```python
from build123d import *

# Parameters (mm, degrees)
F0_R     = 12.7
F0_R_2   = 10.16
F1_DEPTH = 20.32
F2_DEPTH = 20.32
F3_R     = 9.652
F4_DEPTH = 12.7


with BuildPart() as f1:
    # F0 (on Top) → F1 (new body)
    with BuildSketch(Plane.XY):
        with Locations((-39.235822, 31.019291)):
            Circle(F0_R)
        with Locations((-39.235822, 31.019291)):
            Circle(F0_R_2, mode=Mode.SUBTRACT)
    extrude(amount=F1_DEPTH)

    # F0 (on Top) → F2 (join)
    with BuildSketch(Plane.XY):
        with Locations((-39.235822, 31.019291)):
            Circle(F0_R_2)
        Polygon((-40.496945, 38.614266), (-33.288942, 35.908943), (-32.027819, 28.313968), (-37.974699, 23.424316), (-45.182701, 26.129639), (-46.443824, 33.724614), align=None, mode=Mode.SUBTRACT)
    extrude(amount=F2_DEPTH)

    # F3 (on face) → F4 (cut)
    with BuildSketch(Plane(origin=(0, 0, 0), x_dir=(1, 0, 0), z_dir=(0, 0, -1))):
        with Locations((-39.235822, -31.019291)):
            Circle(F3_R)
    extrude(amount=-F4_DEPTH, mode=Mode.SUBTRACT)


solid = f1.part
```
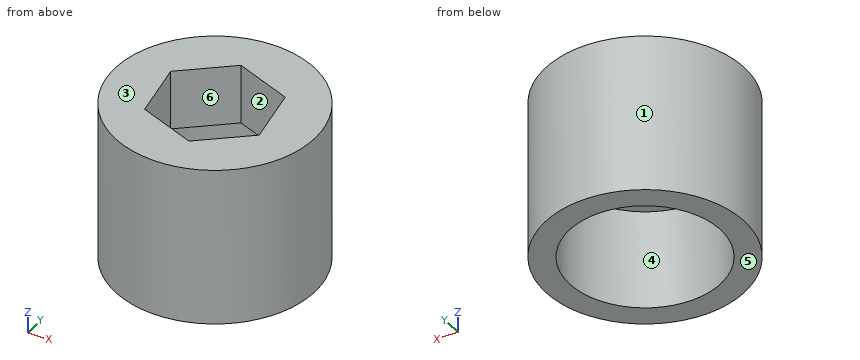
Input: part model. Units: mm. Frame: model coordinates. Face numbers are marked on the shaded views. A direction names the side the tool comes from. Coordinates: 2 decimals unless noted, no trailing zeros. Write each loop counter-clockwise with the first axis right and the second up, starting at its lowest first coordinate (ties: lowest second). Pieces come first, ordered by that corner, then holes. Notation, with made-up numbers: (0, -12) - (14, -12) arc R27 ccw to (14, 8) - close; hole circle Ø10 at (20.25, -39.75). An arc over 180 degrees is marked (long way). Put each result on its own line as item: value. Start each with the question number.
1) Cut plane B-B (x = -37). Return the cut outline in (y, z), plus the area to 3 significant figures.
2) Ray query, L1, parallel to X at y = 25.5, z = 7.25; L2, parallel to Y at x = -39, z = 12.75; L3, parallel to X at y = 33.25, z = 1. Return the intervals inside material, ascending.
3) Cut plane A-A (y = 30.5). Return the cut outline in (x, z), plus the area to 3 significant figures.
4) Cut plane D-D (y = 22.75). Return the cut outline in (x, z).
5) Mould query, pull axis Y, two halves, no side actions, for the marked faces 1, 2 and 3. Classes: pulls with the +Y half, pulls with the -Y half, needs draft (parallel to the pull), parting line crosses it, or undercut.
6) Cut plane C-C (z = 1.75). Return the cut outline in (x, y).
7) Contact query for flat-ended pins moving along their axis: pin 1 (1.5 mm diameter, centred on x = -32, z = 17.5, fed in from -Y); pin 2 (2 mm diameter, centred on y = 22, z = 5.5, fed in from +X); pin 3 (2 mm diameter, centred on x = -41.5, z = 14, fed in from +Y). Output: stop coordinate, or through.
8) Reachability of the marked faces 4, 5 and 6 from +Z, -Z, +X, -X, +Y, -Y: full face, straight path, thin tool, end or side. Return the list, or none.
Resolved:
1. outline: (18.52, 0) - (21.63, 0) - (21.63, 12.7) - (24.23, 12.7) - (24.23, 20.32) - (18.52, 20.32) - close; (37.3, 12.7) - (40.41, 12.7) - (40.41, 0) - (43.52, 0) - (43.52, 20.32) - (37.3, 20.32) - close
1. area: 170 mm2
2. L1: x = -50.67 to -47.15, -31.32 to -27.8
2. L2: y = 18.32 to 23.81, 38.05 to 43.72
2. L3: x = -51.74 to -48.63, -29.85 to -26.73
3. outline: (-51.93, 0) - (-48.87, 0) - (-48.87, 12.7) - (-45.91, 12.7) - (-45.91, 20.32) - (-51.93, 20.32) - close; (-32.39, 12.7) - (-29.6, 12.7) - (-29.6, 0) - (-26.55, 0) - (-26.55, 20.32) - (-32.39, 20.32) - close
3. area: 168 mm2
4. outline: (-48.87, 0) - (-44.21, 0) - (-44.21, 12.7) - (-34.26, 12.7) - (-34.26, 0) - (-29.6, 0) - (-29.6, 20.32) - (-48.87, 20.32) - close
5. face 1: parting line crosses it
5. face 2: undercut
5. face 3: needs draft
6. outline: circle Ø25.4 at (-39.24, 31.02); hole circle Ø19.3 at (-39.24, 31.02)
7. pin 1: stops at y = 20.1
7. pin 2: stops at x = -29.39
7. pin 3: stops at y = 43.66
8. face 4: -Z
8. face 5: -Z, +X, -X, +Y, -Y
8. face 6: +Z, -Z
